Work out the finished part from the listing and answer in its coordinate system (mm). A direction names the side the tool comes from. Round coordinates to 2 decimals unless told otherwise and drop trailing zeros. Write each loop counter-clockwise with the first axis right and the second up, starting at its lowest first coordinate (ties: lowest second). Pieces come first, ordered by that corner, then holes. Notation, with made-up numbers: (83, 45) - (130, 45) arc R19 cw to (130, 61) - close; hole circle Ø3 at (41.25, 16.5). An arc over 180 degrees is marked (long way). Answer as a JSON object with one key per item and string values.
```python
from build123d import *

# Parameters (mm, degrees)
CROQUIS11_W                       = 76.2
CROQUIS11_H                       = 19.05
AL_SOLID_PROFILES_3_X_0_5_1_DEPTH = 93.65
CORTAR_EXTRUIR1_DEPTH             = 103.882627299
DI_METRO_DE_TALADRO_10_0_10_1_D   = 10
TALADRO_ROSCADO_M31_REACH         = 104.883
TALADRO_ROSCADO_M31_BORE_R        = 1.25


with BuildPart() as part:
    # Croquis11 → Al solid profiles 3 X 0.5(1) (new body)
    with BuildSketch(Plane(origin=(0, 93.65, 0), x_dir=(0, 0, 1), z_dir=(0, -1, 0))):
        Rectangle(CROQUIS11_W, CROQUIS11_H)
    extrude(amount=AL_SOLID_PROFILES_3_X_0_5_1_DEPTH)

    # Croquis12 → Cortar-Extruir1 (cut, through all)
    with BuildSketch(Plane(origin=(9.525, 0, 0), x_dir=(0, 0, -1), z_dir=(1, 0, 0))):
        with BuildLine():
            Line((-17.7, 83.65), (-17.7, 68.65))
            ThreePointArc((-17.7, 68.65), (-21, 65.35), (-24.3, 68.65))
            Line((-24.3, 68.65), (-24.3, 83.65))
            ThreePointArc((-24.3, 83.65), (-21, 86.95), (-17.7, 83.65))
        make_face()
        with BuildLine():
            Line((17.7, 83.65), (17.7, 68.65))
            ThreePointArc((17.7, 68.65), (21, 65.35), (24.3, 68.65))
            Line((24.3, 68.65), (24.3, 83.65))
            ThreePointArc((24.3, 83.65), (21, 86.95), (17.7, 83.65))
        make_face()
    extrude(amount=-CORTAR_EXTRUIR1_DEPTH, mode=Mode.SUBTRACT)

    # Diámetro de taladro Ø10.0 (10)1 (through all)
    with Locations(Plane(origin=(0, 0, -38.1), x_dir=(-1, 0, 0), z_dir=(0, 0, -1))):
        with Locations((0, 10)):
            Hole(DI_METRO_DE_TALADRO_10_0_10_1_D / 2)

    # Taladro roscado M31 bore → Taladro roscado M31 (cut, up to next)
    with BuildSketch(Plane(origin=(9.525, 0, 0), x_dir=(0, 0, -1), z_dir=(1, 0, 0)), mode=Mode.PRIVATE) as taladro_roscado_m31_sk1:
        with Locations((20, 10)):
            Circle(TALADRO_ROSCADO_M31_BORE_R)
    taladro_roscado_m31_tool1 = extrude(taladro_roscado_m31_sk1.sketch, amount=-TALADRO_ROSCADO_M31_REACH, mode=Mode.PRIVATE) & part.part
    # Taladro roscado M31 bore → Taladro roscado M31 (cut, up to next)
    with BuildSketch(Plane(origin=(9.525, 0, 0), x_dir=(0, 0, -1), z_dir=(1, 0, 0)), mode=Mode.PRIVATE) as taladro_roscado_m31_sk2:
        with Locations((-20, 10)):
            Circle(TALADRO_ROSCADO_M31_BORE_R)
    taladro_roscado_m31_tool2 = extrude(taladro_roscado_m31_sk2.sketch, amount=-TALADRO_ROSCADO_M31_REACH, mode=Mode.PRIVATE) & part.part
    add(taladro_roscado_m31_tool1.solids().sort_by_distance((9.525, 10, -20))[0], mode=Mode.SUBTRACT)
    add(taladro_roscado_m31_tool2.solids().sort_by_distance((9.525, 10, 20))[0], mode=Mode.SUBTRACT)


solid = part.part
```
Item 1: A cutting plane is placed at B-B (y = 81.5). Write down the section's boundary in (x, z) (3 decimals), and give its area (3 significant figures).
Results found:
{"outline": "(-9.525, -38.1) - (9.525, -38.1) - (9.525, -24.3) - (-9.525, -24.3) - close; (-9.525, -17.7) - (9.525, -17.7) - (9.525, 17.7) - (-9.525, 17.7) - close; (-9.525, 24.3) - (9.525, 24.3) - (9.525, 38.1) - (-9.525, 38.1) - close", "area": "1,200 mm²"}
Item 2: A cutting plane is placed at A-A (x = 0). Write down the section's boundary in (y, z).
Results found:
{"outline": "(0, -38.1) - (5, -38.1) - (5, 38.1) - (0, 38.1) - close; (15, -38.1) - (93.65, -38.1) - (93.65, 38.1) - (15, 38.1) - close; hole (68.65, -24.3) - (83.65, -24.3) arc R3.3 ccw to (83.65, -17.7) - (68.65, -17.7) arc R3.3 ccw to start; hole (68.65, 17.7) - (83.65, 17.7) arc R3.3 ccw to (83.65, 24.3) - (68.65, 24.3) arc R3.3 ccw to start"}
Item 3: A cutting plane is placed at C-C (z = 11). Write down the section's boundary in (x, y) (3 decimals), and give its area (3 significant figures).
Results found:
{"outline": "(-9.525, 0) - (9.525, 0) - (9.525, 93.65) - (-9.525, 93.65) - close; hole circle Ø10 at (0, 10)", "area": "1,710 mm²"}
Item 4: This flat-tipped pin is pushed along its axis until it touches: P1, Ø1, axis at x = 2.5, z = -19.5, coming from the -Y side. Where does it stop, or does it pass through?
Results found:
{"P1": "y = 0"}
Item 5: For faces 1 (the cylindrical face through (7.216, 11.054, -20.672)), 2 (the flat face through (-9.525, 47, -1)), 3 (the flat face through (0, 76, -24.3)), determine the directions among +Z, -Z, +X, -X, +Y, -Y from which every point of the face is accessible in a straight line to the end or side of a thin tool.
Results found:
{"face 1": "+X", "face 2": "+Z, -Z, -X, +Y, -Y", "face 3": "+X, -X"}
Item 6: Determine the mould class of faces 4 (the flat face through (0, 76, -17.7)), 5 (the flat face through (0, 0, -1)), 6 (the flat face through (0, 47, -38.1)) for opening direction Z: pulls with the +Z half, pulls with the -Z half, needs draft (parallel to the pull), parting line crosses it, or undercut.
Results found:
{"face 4": "undercut", "face 5": "needs draft", "face 6": "pulls with the -Z half"}
Item 7: Consider line 1 along Z through (x, y) = (7.05, 10); line 2 along Y through (x, z) = (8.3, 20); line 3 along Y through (x, z) = (0, -3). Determine where each line is inside the solid, lowest interval first.
Results found:
{"line 1": "-38.1 to -21.25, -18.75 to 18.75, 21.25 to 38.1", "line 2": "0 to 8.75, 11.25 to 65.51, 86.79 to 93.65", "line 3": "0 to 5, 15 to 93.65"}
Item 8: A cutting plane is placed at D-D (x = 8.25). Write down the section's boundary in (y, z).
Results found:
{"outline": "(0, -38.1) - (93.65, -38.1) - (93.65, 38.1) - (0, 38.1) - close; hole circle Ø2.5 at (10, -20); hole circle Ø2.5 at (10, 20); hole (68.65, -24.3) - (83.65, -24.3) arc R3.3 ccw to (83.65, -17.7) - (68.65, -17.7) arc R3.3 ccw to start; hole (68.65, 17.7) - (83.65, 17.7) arc R3.3 ccw to (83.65, 24.3) - (68.65, 24.3) arc R3.3 ccw to start"}
